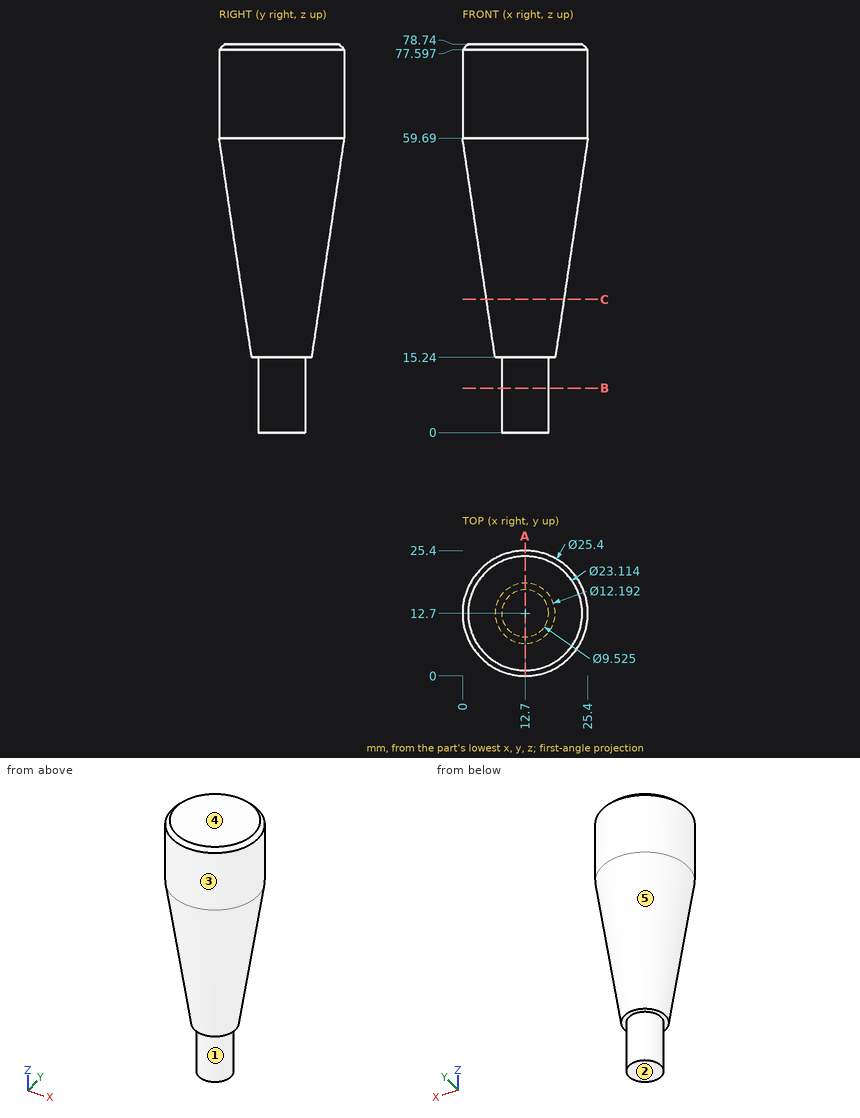
Can you work these out from the drawing? Everything is in mm from the part's minimum corner. A direction names the side the tool comes from. Give positions to 0.01 mm unless a question says otherwise; leave off trailing zeros. Loops run counter-clockwise (first coordinate to the right, second up) from the corner with the lowest first, then second, coordinate; pieces in that order, holes last. Notation, with made-up numbers: M 6,71.5 L 24,71.5 A14 cw 24,92.5 Z; hole C 63,84 d11. An arc over 180 degrees is marked long. Put each result on its own line as item: value. Start each with the question number.
(1) For the marked faces 1 and 2, which set-ups out of +Z, -Z, +X, -X, +Y, -Y let a thin tool reach every point of the face, with its end or its side?
(2) Will these pins go through, and if not, where does the flat tip stop? pin 1 Ø1 at (x, z) = (3, 65) entering from -Y (3 decimals); pin 2 Ø13.5 at (x, y) = (15, 13) entering from -Z; pin 3 Ø3 at (x, z) = (11.5, 44) entering from +Y; pin 4 Ø12 at (x, z) = (22.5, 22) entering from +Y.
(3) I want a section at B-B on z = 9. Please give me the cut outline in (x, y) (1 decimal).
(4) If we mould it in two halves opening along Z, with no side actions, what happens to the marked faces 3, 4 and 5? For each: +Z half, -Z half, draft (parallel to the pull), parting line (faces both ways), or undercut.
(5) I need wall thicknesses on line 1 along X through (y, z) = (13, 68); line 2 along Z through (x, y) = (18.25, 15); line 3 along Y through (x, z) = (13, 40). Which ranges of each line are inside material? Lowest first, please. Write a range as [from, to].
(6) I want a section at A-A on x = 12.7. Please give me the cut outline in (y, z), then the cut area to 3 significant figures.
(7) I want a section at C-C on z = 27. Please give me the cut outline in (x, y), then the cut area to 3 significant figures.
Answer block:
1. face 1: -Z
1. face 2: -Z, +X, -X, +Y, -Y
2. pin 1: y = 3.945
2. pin 2: z = 0
2. pin 3: y = 23.26
2. pin 4: y = 18.84
3. outline: C 12.7,12.7 d9.5
4. face 3: draft
4. face 4: +Z half
4. face 5: -Z half
5. line 1: [0, 25.4]
5. line 2: [15.24, 78.74]
5. line 3: [2.93, 22.47]
6. outline: M 0,59.69 L 6.6,15.24 L 7.94,15.24 L 7.94,0 L 17.46,0 L 17.46,15.24 L 18.8,15.24 L 25.4,59.69 L 25.4,77.6 L 24.26,78.74 L 1.14,78.74 L 0,77.6 Z
6. area: 1,460 mm^2
7. outline: C 12.7,12.7 d15.69
7. area: 193 mm^2
